Design review of the part built by this model. Coordinates are the model's own, in mm. Coordinates: 2 decimals unless noted, no trailing zeros. Loops run counter-clockwise (first coordinate to the right, second up) from the corner with the lowest first, then second, coordinate; pieces in that order, holes last. Notation, with made-up numbers: M -35,59 L -22,59 A22 ccw -22,92 Z; hole C 88.5,11 d4. An arc over 180 degrees is marked long. Put each result on its own line as item: value. Start each with the question number.
(1) Clearance check with a flat-ended pin moving along its axis: pin 1 (13 mm diameter, centred on x = -101.28, y = 175.42, fed in from -Z). State where the tip first meets the part, or that it passes through.
(2) Take a section at C-C, the plane y = 55. Give the boundary of the cut face in (x, z), then the cut area to 3 significant figures.
(3) For probe 1 along Y at (x, z) = (-143, 1.7); probe 2 along X at (y, z) = (-55, 1.2); probe 3 along X at (y, z) = (101, 2), list the stretches that pass through material, from the lowest coordinate up. Write a range as [from, to].
(4) Take a section at B-B, the plane z = 1.1. Count the separate pieces of the cut face and the enclosed holes in it, then the cut area to 3 significant figures.
(5) Take a section at A-A, the plane y = 0. Give the boundary of the cut face in (x, z).
(6) Take a section at D-D, the plane x = -157. Give the boundary of the cut face in (y, z).
```python
from build123d import *

# Parameters (mm, degrees)
SKETCH1_R               = 250
BOSS_EXTRUDE1_DEPTH     = 4
CUT_EXTRUDE7_DEPTH      = 354.576017286
CUT_EXTRUDE7_DEPTH_BACK = 354.576017286
SKETCH12_R              = 6.1
SKETCH12_R_2            = 7.5
SKETCH12_R_3            = 6
SKETCH12_R_4            = 4.1


with BuildPart() as part:
    # Sketch1 → Boss-Extrude1 (new body)
    with BuildSketch(Plane.XY):
        Circle(SKETCH1_R)
    extrude(amount=BOSS_EXTRUDE1_DEPTH)

    # Sketch12 → Cut-Extrude7 (cut, two sides: drawn at the far end of the back side and taken through both)
    with BuildSketch(Plane.XY.offset(4).offset(-CUT_EXTRUDE7_DEPTH_BACK)):
        with Locations((-141.238075794, 55)):
            Circle(SKETCH12_R)
        with Locations((-106.238075794, 0)):
            Circle(SKETCH12_R_2)
        with Locations((106.238075794, 0)):
            Circle(SKETCH12_R_2)
        with Locations((-141.238075794, -55)):
            Circle(SKETCH12_R_3)
        with Locations((141.238075794, -55)):
            Circle(SKETCH12_R_3)
        with Locations((141.238075794, 55)):
            Circle(SKETCH12_R_3)
        with Locations((0, -202.556165051)):
            Circle(SKETCH12_R_4)
        with Locations((-52.425393218, -195.654231096)):
            Circle(SKETCH12_R_4)
        with Locations((-101.278082525, -175.418784627)):
            Circle(SKETCH12_R_4)
        with Locations((-143.228837878, -143.228837878)):
            Circle(SKETCH12_R_4)
        with Locations((-175.418784627, -101.278082525)):
            Circle(SKETCH12_R_4)
        with Locations((-175.418784627, 101.278082525)):
            Circle(SKETCH12_R_4)
        with Locations((-143.228837878, 143.228837878)):
            Circle(SKETCH12_R_4)
        with Locations((-101.278082525, 175.418784627)):
            Circle(SKETCH12_R_4)
        with Locations((-52.425393218, 195.654231096)):
            Circle(SKETCH12_R_4)
        with Locations((0, 202.556165051)):
            Circle(SKETCH12_R_4)
        with Locations((52.425393218, 195.654231096)):
            Circle(SKETCH12_R_4)
        with Locations((101.278082525, 175.418784627)):
            Circle(SKETCH12_R_4)
        with Locations((143.228837878, 143.228837878)):
            Circle(SKETCH12_R_4)
        with Locations((175.418784627, 101.278082525)):
            Circle(SKETCH12_R_4)
        with Locations((175.418784627, -101.278082525)):
            Circle(SKETCH12_R_4)
        with Locations((143.228837878, -143.228837878)):
            Circle(SKETCH12_R_4)
        with Locations((101.278082525, -175.418784627)):
            Circle(SKETCH12_R_4)
        with Locations((52.425393218, -195.654231096)):
            Circle(SKETCH12_R_4)
    extrude(amount=CUT_EXTRUDE7_DEPTH + CUT_EXTRUDE7_DEPTH_BACK, mode=Mode.SUBTRACT)


solid = part.part
```
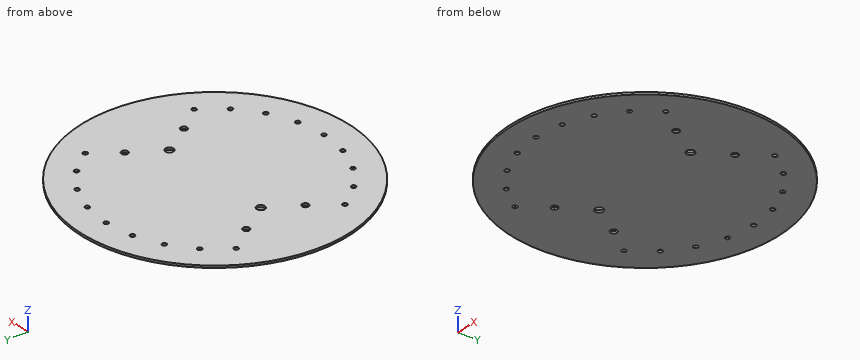
Computed values:
1. pin 1: stops at z = 0
2. outline: M -243.87,0 L -147.34,0 L -147.34,4 L -243.87,4 Z; M -135.14,0 L 135.24,0 L 135.24,4 L -135.14,4 Z; M 147.24,0 L 243.87,0 L 243.87,4 L 147.24,4 Z
2. area: 1,850 mm^2
3. probe 1: y = [-205.06, -147.32], [-139.14, -60.74], [-49.26, 49.16], [60.84, 139.14], [147.32, 205.06]
3. probe 2: x = [-243.87, -147.24], [-135.24, 135.24], [147.24, 243.87]
3. probe 3: x = [-228.69, -179.51], [-171.33, 171.33], [179.51, 228.69]
4. separate pieces: 1
4. enclosed holes: 24
4. area: 195,000 mm^2
5. outline: M -250,0 L -113.74,0 L -113.74,4 L -250,4 Z; M -98.74,0 L 98.74,0 L 98.74,4 L -98.74,4 Z; M 113.74,0 L 250,0 L 250,4 L 113.74,4 Z
6. outline: M -194.55,0 L 194.55,0 L 194.55,4 L -194.55,4 Z
